Geometry check sheet. Reference: the model listing, model coordinates, mm. A direction names the side the tool comes from. Coordinates: 2 decimals unless noted, no trailing zeros. Order: outer loops, then holes, each group sorted by start corner. A loop starts at its lowest first (then second) coordinate and runs counter-clockwise, first axis right, second up. Notation, with made-up numbers: (-20.5, -39) - (4.5, -39) arc R15 cw to (4.5, -35) - close; hole circle Ø5 at (22.25, -17.5). An arc over 180 degrees is marked (long way). Put each result on its own line as item: value.
from build123d import *

# Parameters (mm, degrees)
SKETCH1_W          = 15.875
SKETCH1_H          = 2.413
CHAMFER1_SIZE      = 0.5953125
CUT_EXTRUDE2_DEPTH = 1.79578
SKETCH6_R          = 1.833087105
CUT_EXTRUDE3_DEPTH = 1.79578
CUT_EXTRUDE3_TAPER = 45


with BuildPart() as part:
    # Sketch1 → Revolve1 (revolve)
    with BuildSketch(Plane(origin=(0, 0, 0), x_dir=(0, 0, -1), z_dir=(1, 0, 0))):
        with Locations((10.5029, 1.2065)):
            Rectangle(SKETCH1_W, SKETCH1_H)
    revolve(axis=Axis((0, 0, -18.4404), (0, 0, 1)))

    # Chamfer1
    chamfer1_edges = [part.edges().sort_by_distance(p)[0] for p in [
        (0, -2.413, -18.4404),
    ]]
    chamfer(chamfer1_edges, length=CHAMFER1_SIZE)

    # Sketch7 → Revolve2 (revolve)
    with BuildSketch(Plane(origin=(0, 0, 0), x_dir=(0, 0, -1), z_dir=(1, 0, 0)), mode=Mode.PRIVATE) as revolve2_sk:
        with BuildLine():
            Line((2.18059, 4.5847), (2.5654, 4.5847))
            Line((2.5654, 4.5847), (2.5654, 0))
            Line((2.5654, 0), (0, 0))
            Line((0, 0), (0, 2.413))
            ThreePointArc((0, 2.413), (0.925030326, 3.664791196), (2.18059, 4.5847))
        make_face()
    revolve(revolve2_sk.sketch.rotate(Axis((0, 0, 0), (0, 0, -1)), 180), axis=Axis((0, 0, 0), (0, 0, -1)))

    # Sketch5 → Cut-Extrude2 (cut)
    with BuildSketch(Plane.XY):
        Polygon((1.5875, -0.916543552), (1.5875, 0.916543552), (0, 1.833087105), (-1.5875, 0.916543552), (-1.5875, -0.916543552), (0, -1.833087105), align=None)
    extrude(amount=-CUT_EXTRUDE2_DEPTH, mode=Mode.SUBTRACT)

    # Sketch6 → Cut-Extrude3 (cut)
    with BuildSketch(Plane.XY):
        Circle(SKETCH6_R)
    extrude(amount=-CUT_EXTRUDE3_DEPTH, taper=CUT_EXTRUDE3_TAPER, mode=Mode.SUBTRACT)


solid = part.part
Q1. Depth check by flat-ended pin: pin 1 Ø5 at (x, z) = (-2, -8.5) entering from -Y; pin 2 Ø2 at (y, z) = (0, -0.5) entering from +X; pin 3 Ø1 at (y, z) = (-2, -9.5) entering from +X. Enter the tip coordinate at first touch or a pass-through.
Answer block:
pin 1: stops at y = -2.41
pin 2: stops at x = 4.16
pin 3: stops at x = 1.89
Q2. Access from +Z, -Z, +X, -X, +Y, -Y to the whole of each face (thin tool, end or side, straight path). Record for faces 1 (the cylindrical face through (1.468, -1.915, -10.312)), 2 (the flat face through (0.8, 1.37, -0.89)), 3 (the flat face through (0, 0, -18.44)).
Answer block:
face 1: -Z
face 2: +Z
face 3: -Z, +X, -X, +Y, -Y
Q3. Thickness scan on L1, parallel to Z at x = 1, y = -1; L2, parallel to Z at x = 2.25, y = 3.75; L3, parallel to X at y = 2, z = -1.25. Record the ranges inside material, lowest first. Write a range as [from, to].
Answer block:
L1: z = [-18.44, -1.8]
L2: z = [-2.57, -1.81]
L3: x = [-3.42, 3.42]
Q4. Draft check along Y on faces 4 (the flat face through (-0.8, -1.37, -0.89)), 5 (the cylindrical face through (4.476, 0.994, -2.376)), 6 (the flat face through (2, -2, -2.565)). Enter one of: pulls with the +Y half, pulls with the -Y half, needs draft (parallel to the pull), parting line crosses it, or undercut.
Answer block:
face 4: undercut
face 5: parting line crosses it
face 6: needs draft
Q5. Section check B-B on z = -14. Record the boundary of the cut face in (x, y), then the cut area to 3 significant figures.
Answer block:
outline: circle Ø4.83 at (0, 0)
area: 18.3 mm^2
Q6. Section check A-A on y = 0. Record the boundary of the cut face in (x, z).
Answer block:
outline: (-4.58, -2.57) - (-2.41, -2.57) - (-2.41, -17.85) - (-1.82, -18.44) - (1.82, -18.44) - (2.41, -17.85) - (2.41, -2.57) - (4.58, -2.57) - (4.58, -2.18) arc R5.17 ccw to (2.41, 0) - (1.83, 0) - (1.59, -0.25) - (1.59, -1.8) - (-1.59, -1.8) - (-1.59, -0.25) - (-1.83, 0) - (-2.41, 0) arc R5.17 ccw to (-4.58, -2.18) - close
